CAD build for the part. Positions are in the model's coordinates, mm. Give positions to 0.01 mm unless a question says otherwise; leave off trailing zeros. Write each loop counter-clockwise with the first axis right and the second up, starting at its lowest first coordinate (ties: lowest second). Pieces come first, ordered by that corner, then holes. Notation, with made-up numbers: (57, 29) - (87, 29) arc R17 ccw to (87, 61) - close; hole circle Ø3 at (48.5, 68.5). An arc over 180 degrees is marked (long way). Answer as a JSON object with one key per item and string values.
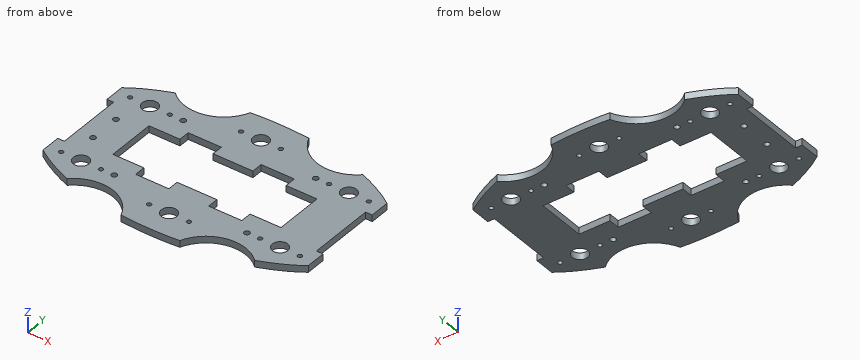
from build123d import *

# Parameters (mm, degrees)
SKETCH1_RX          = 75
SKETCH1_RY          = 40
SKETCH1_R           = 3.5
BOSS_EXTRUDE1_DEPTH = 3
SKETCH2_R           = 1.25
SKETCH2_R_2         = 18
CUT_EXTRUDE1_DEPTH  = 10
SKETCH4_R           = 1
CUT_EXTRUDE2_DEPTH  = 10
SKETCH9_R           = 1.25
CUT_EXTRUDE3_DEPTH  = 3


with BuildPart() as part:
    # Sketch1 → Boss-Extrude1 (new body)
    with BuildSketch(Plane.XY):
        with Locations((0, 0)):
            Ellipse(SKETCH1_RX, SKETCH1_RY)
        with Locations((0, 28)):
            Circle(SKETCH1_R, mode=Mode.SUBTRACT)
        with Locations((0, -28)):
            Circle(SKETCH1_R, mode=Mode.SUBTRACT)
        with Locations((45, 21)):
            Circle(SKETCH1_R, mode=Mode.SUBTRACT)
        with Locations((-45, 21)):
            Circle(SKETCH1_R, mode=Mode.SUBTRACT)
        with Locations((-45, -21)):
            Circle(SKETCH1_R, mode=Mode.SUBTRACT)
        with Locations((45, -21)):
            Circle(SKETCH1_R, mode=Mode.SUBTRACT)
    extrude(amount=BOSS_EXTRUDE1_DEPTH)

    # Sketch2 → Cut-Extrude1 (cut)
    with BuildSketch(Plane.XY.offset(3)):
        with Locations((-30, 21)):
            Circle(SKETCH2_R)
        with Locations((30, 21)):
            Circle(SKETCH2_R)
        with Locations((30, -21)):
            Circle(SKETCH2_R)
        with Locations((-30, -21)):
            Circle(SKETCH2_R)
        with Locations((30, 46)):
            Circle(SKETCH2_R_2)
        with Locations((-30, 46)):
            Circle(SKETCH2_R_2)
        with Locations((30, -46)):
            Circle(SKETCH2_R_2)
        with Locations((-30, -46)):
            Circle(SKETCH2_R_2)
        with BuildLine():
            Line((60, 24), (60, 15))
            Line((60, 15), (57, 15))
            Line((57, 15), (57, -15))
            Line((57, -15), (60, -15))
            Line((60, -15), (60, -24))
            add(Edge.make_bspline(
                [(60, -24), (93.75, 0), (60, 24)],
                knots=[5.639684198, 5.639684198, 5.639684198, 6.926686416, 6.926686416, 6.926686416], degree=2, weights=[1, 0.8, 1]))
        make_face()
        with BuildLine():
            Line((-60, 24), (-60, 15))
            Line((-60, 15), (-57, 15))
            Line((-57, 15), (-57, -15))
            Line((-57, -15), (-60, -15))
            Line((-60, -15), (-60, -24))
            add(Edge.make_bspline(
                [(-60, 24), (-93.75, 0), (-60, -24)],
                knots=[2.498091545, 2.498091545, 2.498091545, 3.785093762, 3.785093762, 3.785093762], degree=2, weights=[1, 0.8, 1]))
        make_face()
    extrude(amount=-CUT_EXTRUDE1_DEPTH, mode=Mode.SUBTRACT)

    # Sketch4 → Cut-Extrude2 (cut)
    with BuildSketch(Plane.XY.offset(3)):
        with Locations((9, 28)):
            Circle(SKETCH4_R)
        with Locations((-9, 28)):
            Circle(SKETCH4_R)
        with Locations((9, -28)):
            Circle(SKETCH4_R)
        with Locations((-9, -28)):
            Circle(SKETCH4_R)
        with Locations((54, 21)):
            Circle(SKETCH4_R)
        with Locations((36, 21)):
            Circle(SKETCH4_R)
        with Locations((54, -21)):
            Circle(SKETCH4_R)
        with Locations((36, -21)):
            Circle(SKETCH4_R)
        with Locations((-36, 21)):
            Circle(SKETCH4_R)
        with Locations((-54, 21)):
            Circle(SKETCH4_R)
        with Locations((-36, -21)):
            Circle(SKETCH4_R)
        with Locations((-54, -21)):
            Circle(SKETCH4_R)
        Polygon((-9, 11), (9, 11), (9, 16), (24, 16), (24, 11), (38, 11), (38, -11), (24, -11), (24, -16), (9, -16), (9, -11), (-9, -11), (-9, -16), (-24, -16), (-24, -11), (-38, -11), (-38, 11), (-24, 11), (-24, 16), (-9, 16), align=None)
    extrude(amount=-CUT_EXTRUDE2_DEPTH, mode=Mode.SUBTRACT)

    # Sketch9 → Cut-Extrude3 (cut)
    with BuildSketch(Plane(origin=(0, 0, 0), x_dir=(-1, 0, 0), z_dir=(0, 0, -1))):
        with Locations((50, 7)):
            Circle(SKETCH9_R)
        with Locations((50, -7)):
            Circle(SKETCH9_R)
    extrude(amount=-CUT_EXTRUDE3_DEPTH, mode=Mode.SUBTRACT)


solid = part.part
Item 1: Probe line 1 (Y direction, x = 0, z = 1.35); line 2 (X direction, y = 31, z = 1.15); line 3 (Y direction, x = -44, z = 2.15). List the from-to ranges inside material, lowest first. Write a range as from..to.
Entries:
{"line 1": "-40..-31.5, -24.5..-11, 11..24.5, 31.5..40", "line 2": "-47.4..-39.95, -20.05..-1.8, 1.8..20.05, 39.95..47.4", "line 3": "-32.39..-24.35, -17.65..17.65, 24.35..32.39"}
Item 2: Flat gauge pins, fed straight in: P1, Ø1.2, axis at x = -36, y = 21, coming from the -Z side; P2, Ø1, axis at y = -3.5, z = 1, coming from the +X side; P3, Ø0.9, axis at x = -58, z = 1, coming from the +Y side. Where does each tip first touch, or does it go through?
Entries:
{"P1": "through", "P2": "x = 57", "P3": "y = 25.65"}
Item 3: Cut at C-C (x = 45). State how many separate pieces and enclosed holes the cut face has, and give its area (3 significant figures).
Entries:
{"separate pieces": "3", "enclosed holes": "0", "area": "150 mm2"}
Item 4: Cut at B-B (y = -1.5). Give the cut face in (x, z).
Entries:
{"outline": "(-57, 0) - (-38, 0) - (-38, 3) - (-57, 3) - close; (38, 0) - (57, 0) - (57, 3) - (38, 3) - close"}
Item 5: Cut at A-A (x = -30). Give the cut face in (y, z), and give its area (3 significant figures).
Entries:
{"outline": "(-28, 0) - (-22.25, 0) - (-22.25, 3) - (-28, 3) - close; (-19.75, 0) - (-11, 0) - (-11, 3) - (-19.75, 3) - close; (11, 0) - (19.75, 0) - (19.75, 3) - (11, 3) - close; (22.25, 0) - (28, 0) - (28, 3) - (22.25, 3) - close", "area": "87.0 mm2"}
